```python
from build123d import *

# Parameters (mm, degrees)
SKETCH_1_R          = 6
EXTRUDE_1_DEPTH     = 1
SKETCH_2_W          = 3
SKETCH_2_H          = 3
SKETCH_2_W_2        = 5
SKETCH_2_H_2        = 1
EXTRUDE_2_DEPTH     = 0.8
SKETCH_2_6_W        = 1
SKETCH_2_6_H        = 0.5
SKETCH_2_6_W_2      = 5
SKETCH_2_6_H_2      = 1
EXTRUDE_3_DEPTH     = 0.5
SKETCH_4_W          = 5
SKETCH_4_H          = 5
EXTRUDE_4_DEPTH     = 1
CUT_EXTRUDE_1_REACH = 10.718
SKETCH_5_R          = 0.5


with BuildPart() as part:
    # Sketch 1 → Extrude 1 (new body)
    with BuildSketch(Plane(origin=(0, 0, 0), x_dir=(1, 0, 0), z_dir=(0, 1, 0))):
        with Locations(Location((0, 0, 0), (0, 0, 270))):
            Circle(SKETCH_1_R)
    extrude(amount=EXTRUDE_1_DEPTH)

    # Sketch 2 → Extrude 2 (add)
    with BuildSketch(Plane(origin=(0, 1, 0), x_dir=(1, 0, 0), z_dir=(0, 1, 0))):
        with Locations((1.75, 0)):
            Rectangle(SKETCH_2_W, SKETCH_2_H)
        with Locations((-1.75, 0)):
            Rectangle(SKETCH_2_W, SKETCH_2_H)
        with Locations((0, -4.5)):
            Rectangle(SKETCH_2_W_2, SKETCH_2_H_2)
    extrude(amount=EXTRUDE_2_DEPTH)

    # Sketch 2_6 → Extrude 3 (add)
    with BuildSketch(Plane(origin=(0, 1, 0), x_dir=(1, 0, 0), z_dir=(0, 1, 0))):
        with Locations((-0.75, 3.7)):
            Rectangle(SKETCH_2_6_W, SKETCH_2_6_H)
        with Locations((0.75, 3.7)):
            Rectangle(SKETCH_2_6_W, SKETCH_2_6_H)
        with Locations((0, -4.5)):
            Rectangle(SKETCH_2_6_W_2, SKETCH_2_6_H_2)
    extrude(amount=EXTRUDE_3_DEPTH)

    # Sketch 4 → Extrude 4 (add)
    with BuildSketch(Plane.XZ):
        Rectangle(SKETCH_4_W, SKETCH_4_H)
    extrude(amount=EXTRUDE_4_DEPTH)

    # Sketch 5 → Cut-Extrude 1 (cut, up to next)
    with BuildSketch(Plane(origin=(0, 1, 0), x_dir=(1, 0, 0), z_dir=(0, 1, 0)), mode=Mode.PRIVATE) as cut_extrude_1_sk1:
        with Locations(Location((5, 0, 0), (0, 0, 270))):
            Circle(SKETCH_5_R)
    cut_extrude_1_tool1 = extrude(cut_extrude_1_sk1.sketch, amount=-CUT_EXTRUDE_1_REACH, mode=Mode.PRIVATE) & part.part
    # Sketch 5 → Cut-Extrude 1 (cut, up to next)
    with BuildSketch(Plane(origin=(0, 1, 0), x_dir=(1, 0, 0), z_dir=(0, 1, 0)), mode=Mode.PRIVATE) as cut_extrude_1_sk2:
        with Locations(Location((-5, 0, 0), (0, 0, 270))):
            Circle(SKETCH_5_R)
    cut_extrude_1_tool2 = extrude(cut_extrude_1_sk2.sketch, amount=-CUT_EXTRUDE_1_REACH, mode=Mode.PRIVATE) & part.part
    add(cut_extrude_1_tool1.solids().sort_by_distance((5, 1, 0))[0], mode=Mode.SUBTRACT)
    add(cut_extrude_1_tool2.solids().sort_by_distance((-5, 1, 0))[0], mode=Mode.SUBTRACT)


solid = part.part
```
Work out the finished part from the listing and answer in its coordinate system (mm). A direction names the side the tool comes from. Coordinates: 2 decimals unless noted, no trailing zeros. Loops run counter-clockwise (first coordinate to the right, second up) from the corner with the lowest first, then second, coordinate; pieces in that order, holes last. Notation, with made-up numbers: M 46,59.25 L 57,59.25 A15 cw 57,87.25 Z; hole C 66,-12 d6. An arc over 180 degrees is marked long. Use CSV: the item, a comma, the result in double quotes. Start each with the question number.
(1) Find section A-A, the plane z = 0. Give the vertices of the cut face in (x, y), then the cut area to 3 significant figures.
(2) For faces 1 (the face through (-2.5, -0.5, 0)), 2 (the face through (0, -1, 0)), 3 (the face through (0, -0.5, 2.5)), 4 (the face through (0, -0.5, -2.5)), 5 (the face through (2.5, -0.5, 0)), determine the directions among +Z, -Z, +X, -X, +Y, -Y from which every point of the face is accessible in a straight line to the end or side of a thin tool.
(3) Find section D-D, the plane y = 0.65. Give the vertices of the cut face in (x, z).
(4) For a pull along X with two mould halves and no side action, classify faces 6 (the face through (2, 1.8, 0)), 7 (the face through (1.802, 0.493, 5.723)), 8 (the face through (5.496, 0.507, -0.065)) as +X half, -X half, draft (parallel to the pull), parting line (faces both ways), or undercut.
(5) Consider line 1 (X direction, y = 0.3, z = 0); line 2 (Y direction, x = -5, z = -2.5); line 3 (Y direction, x = -1, z = 2). Determine where each line is inside the solid, lowest interval first.
(6) Find section C-C, the plane x = -5. Give the vertices of the cut face in (y, z).
(7) Given pin 1 Ø0.8 at (y, z) = (-0.5, -1) entering from +X; pin 2 Ø0.6 at (x, y) = (1.5, 1.5) entering from +Z; pin 3 Ø0.9 at (y, z) = (1.5, 0) entering from -X, each flat-ended and moving along its own axis, determine where each tip first touches the part or whether it passes through.
(8) Find section B-B, the plane x = 0. Give the vertices of the cut face in (y, z), then the cut area to 3 significant figures.
Recorded:
1,outline,"M -6,0 L -5.5,0 L -5.5,1 L -6,1 Z; M -4.5,0 L -2.5,0 L -2.5,-1 L 2.5,-1 L 2.5,0 L 4.5,0 L 4.5,1 L 3.25,1 L 3.25,1.8 L 0.25,1.8 L 0.25,1 L -0.25,1 L -0.25,1.8 L -3.25,1.8 L -3.25,1 L -4.5,1 Z; M 5.5,0 L 6,0 L 6,1 L 5.5,1 Z"
1,area,"19.8 mm^2"
2,face 1,"+Z, -Z, -X, -Y"
2,face 2,"+Z, -Z, +X, -X, -Y"
2,face 3,"+Z, +X, -X, -Y"
2,face 4,"-Z, +X, -X, -Y"
2,face 5,"+Z, -Z, +X, -Y"
3,outline,"C 0,0 d12; hole C -5,0 d1; hole C 5,0 d1"
4,face 6,"draft"
4,face 7,"parting line"
4,face 8,"undercut"
5,line 1,"x = -6 to -5.5, -4.5 to 4.5, 5.5 to 6"
5,line 2,"y = 0 to 1"
5,line 3,"y = -1 to 1"
6,outline,"M 0,-3.32 L 1,-3.32 L 1,-0.5 L 0,-0.5 Z; M 0,0.5 L 1,0.5 L 1,3.32 L 0,3.32 Z"
7,pin 1,"stops at x = 2.5"
7,pin 2,"stops at z = 5"
7,pin 3,"stops at x = -3.25"
8,outline,"M -1,-2.5 L 0,-2.5 L 0,-6 L 1,-6 L 1,4 L 1.8,4 L 1.8,5 L 1,5 L 1,6 L 0,6 L 0,2.5 L -1,2.5 Z"
8,area,"17.8 mm^2"
